```python
from build123d import *

# Parameters (mm, degrees)
SKETCH1_R           = 26.162
BOSS_EXTRUDE1_DEPTH = 94.742
SKETCH2_R           = 25.4
CUT_EXTRUDE1_DEPTH  = 35.052
SKETCH3_R           = 20.066
CUT_EXTRUDE2_DEPTH  = 134.62
SKETCH6_W           = 64.219899477
SKETCH6_H           = 22.849587553
CUT_EXTRUDE4_DEPTH  = 33.909
BOSS_EXTRUDE3_DEPTH = 22.86
BOSS_EXTRUDE4_DEPTH = 3.556
FILLET3_R           = 2.54
FILLET4_R           = 0.254


with BuildPart() as part:
    # Sketch1 → Boss-Extrude1 (new body)
    with BuildSketch(Plane.XY):
        Circle(SKETCH1_R)
    extrude(amount=BOSS_EXTRUDE1_DEPTH)

    # Sketch2 → Cut-Extrude1 (cut)
    with BuildSketch(Plane.XY.offset(94.742)):
        with Locations((0, -5.334)):
            Circle(SKETCH2_R)
    extrude(amount=-CUT_EXTRUDE1_DEPTH, mode=Mode.SUBTRACT)

    # Sketch3 → Cut-Extrude2 (cut)
    with BuildSketch(Plane.XY.offset(59.69)):
        with Locations((0, -3.339145452)):
            Circle(SKETCH3_R)
    extrude(amount=-CUT_EXTRUDE2_DEPTH, mode=Mode.SUBTRACT)

    # Sketch6 → Cut-Extrude4 (cut, symmetric)
    with BuildSketch(Plane(origin=(0, 0, 0), x_dir=(0, 0, -1), z_dir=(1, 0, 0))):
        with Locations((-27.580050262, -17.774793777)):
            Rectangle(SKETCH6_W, SKETCH6_H)
    extrude(amount=CUT_EXTRUDE4_DEPTH, both=True, mode=Mode.SUBTRACT)

    # Sketch11 → Boss-Extrude3 (add)
    with BuildSketch(Plane(origin=(0, 0, 0), x_dir=(-1, 0, 0), z_dir=(0, 0, -1))):
        with BuildLine():
            Line((-8.957907595, 23.105072639), (8.957907595, 23.105072639))
            ThreePointArc((8.957907595, 23.105072639), (9.855933208, 22.733098251), (10.227907595, 21.835072639))
            Line((10.227907595, 21.835072639), (10.227907595, 20.473507992))
            ThreePointArc((10.227907595, 20.473507992), (9.855933208, 19.57548238), (8.957907595, 19.203507992))
            Line((8.957907595, 19.203507992), (-8.957907595, 19.203507992))
            ThreePointArc((-8.957907595, 19.203507992), (-9.855933208, 19.57548238), (-10.227907595, 20.473507992))
            Line((-10.227907595, 20.473507992), (-10.227907595, 21.835072639))
            ThreePointArc((-10.227907595, 21.835072639), (-9.855933208, 22.733098251), (-8.957907595, 23.105072639))
        make_face()
    extrude(amount=BOSS_EXTRUDE3_DEPTH)

    # Sketch12 → Boss-Extrude4 (add)
    with BuildSketch(Plane(origin=(0, 0, -22.86), x_dir=(-1, 0, 0), z_dir=(0, 0, -1))):
        with BuildLine():
            Line((-8.539617395, 19.203507992), (8.539617395, 19.203507992))
            ThreePointArc((8.539617395, 19.203507992), (0, 10.663890596), (-8.539617395, 19.203507992))
        make_face()
    extrude(amount=-BOSS_EXTRUDE4_DEPTH)

    # Fillet3
    fillet3_edges = [part.edges().sort_by_distance(p)[0] for p in [
        (0, 19.203507992, -19.304),
    ]]
    fillet(fillet3_edges, radius=FILLET3_R)

    # Fillet4
    fillet4_edges = [part.edges().sort_by_distance(p)[0] for p in [
        (8.539617395, 19.203507992, -19.812),
        (-8.539617395, 19.203507992, -19.812),
    ]]
    fillet(fillet4_edges, radius=FILLET4_R)


solid = part.part
```
Here's how the part is built. I have some questions about the finished solid (model axes, mm). A direction names the side the tool comes from. Give positions to 0.01 mm unless a question says otherwise; leave off trailing zeros. Loops run counter-clockwise (first coordinate to the right, second up) from the corner with the lowest first, then second, coordinate; pieces in that order, holes last. Notation, with made-up numbers: (-9.5, 34.25) -> (30.5, 34.25) arc R17 ccw to (30.5, 64.25) -> close; hole circle Ø4 at (12, 38.5). An arc over 180 degrees is marked (long way). Use one line per item in the form item = value. Start each with the question number.
1) Thinking about a two-plate mould opening in X: for faces 5 (the face through (0.57, 20.06, 77.46)), 6 (the face through (-0.184, 10.666, -20.949)), 7 (the face through (2, 17, 0)), which applies, +X half, -X half, draft (parallel to the pull), parting line (faces both ways), or undercut?
2) Imagine slicing it at C-C (x = 0). Please give me the cut outline in (y, z).
3) Imagine slicing it at D-D (y = 9). Please give me the cut outline in (x, z), then the cut area to 3 significant figures.
4) Imagine slicing it at A-A (y = 0). Please give me the cut outline in (x, z), then the cut area to 3 significant figures.
5) For P1, Ø0.7, axis at y = 21.5, z = -14, coming from the +X side; P2, Ø12, axis at x = 15, y = 2, coming from the -Z side; P3, Ø1, axis at y = 4.5, z = 36.5, coming from the +X side; P4, Ø16.5, axis at x = -2.5, y = 7, coming from the -Z side, each with a flat end and sliding along its axis, tell me the tip position at first contact or that it passes through.
6) Please list where these lines run through material, in increasing order: line 1 along Z through (x, y) = (15.5, 19.5); line 2 along Y through (x, z) = (-9, -7); line 3 along X through (y, z) = (11, 41).
7) Which directions (+Z, -Z, +X, -X, +Y, -Y) give clear straight access to the entire face, cutting with the end or side of a thin tool? Please do faces 1 (the face through (0.48, 16.72, 30.26)), 2 (the face through (-0.12, 18.48, -18.54)), 3 (the face through (2, 17, 59.69)), 4 (the face through (0, 23.105, -11)).
8) Imagine slicing it at B-B (z = -6). Please give me the cut outline in (x, y), then the cut area to 3 significant figures.
Check values:
q1.face_5 = undercut
q1.face_6 = parting line
q1.face_7 = draft
q2.outline = (10.66, -22.86) -> (23.11, -22.86) -> (23.11, 0) -> (26.16, 0) -> (26.16, 94.74) -> (20.07, 94.74) -> (20.07, 59.69) -> (16.73, 59.69) -> (16.73, 0) -> (19.2, 0) -> (19.2, -16.76) arc R2.54 cw to (16.66, -19.3) -> (10.66, -19.3) -> close
q3.outline = (-24.57, 0) -> (-15.82, 0) -> (-15.82, 59.69) -> (-20.97, 59.69) -> (-20.97, 94.74) -> (-24.57, 94.74) -> close; (15.82, 0) -> (24.57, 0) -> (24.57, 94.74) -> (20.97, 94.74) -> (20.97, 59.69) -> (15.82, 59.69) -> close
q3.area = 1,300 mm^2
q4.outline = (-26.16, 0) -> (-19.79, 0) -> (-19.79, 59.69) -> (-24.83, 59.69) -> (-24.83, 94.74) -> (-26.16, 94.74) -> close; (19.79, 0) -> (26.16, 0) -> (26.16, 94.74) -> (24.83, 94.74) -> (24.83, 59.69) -> (19.79, 59.69) -> close
q4.area = 854 mm^2
q5.P1 = 10.23
q5.P2 = 0
q5.P3 = 25.85
q5.P4 = -22.86
q6.line_1 = 0 to 94.74
q6.line_2 = 19.2 to 23.1
q6.line_3 = -23.74 to -14.04, 14.04 to 23.74
q7.face_1 = +Z
q7.face_2 = +X, -X, -Y
q7.face_3 = +Z, -Y
q7.face_4 = -Z, +X, -X, +Y
q8.outline = (-10.23, 20.47) arc R1.27 ccw to (-8.96, 19.2) -> (8.96, 19.2) arc R1.27 ccw to (10.23, 20.47) -> (10.23, 21.84) arc R1.27 ccw to (8.96, 23.11) -> (-8.96, 23.11) arc R1.27 ccw to (-10.23, 21.84) -> close
q8.area = 78.4 mm^2
